Here's how the part is built. I have some questions about the finished solid (model axes, mm). A direction names the side the tool comes from. Coordinates: 2 decimals unless noted, no trailing zeros. Order: outer loops, then holes, each group sorted by start corner. A loop starts at its lowest first (then second) coordinate and runs counter-clockwise, first axis right, second up. Notation, with made-up numbers: (-27.5, -32.75) - (-9.5, -32.75) arc R7 ccw to (-9.5, -21.75) - close; hole circle Ø9 at (89.5, 31). An arc over 180 degrees is marked (long way). Answer as CSV lines item,"result". Start each with the question number.
Q1. I need wall thicknesses on line 1 (Z direction, x = 0, y = 63); line 2 (Y direction, x = -1.25, z = -1). Which ranges of each line are inside material? Lowest first, please.
Q2. Suppose I cut it at C-C (y = 25). Please give me the cut outline in (x, z).
Q3. Suppose I cut it at A-A (y = 59.5). Please give me the cut outline in (x, z), then the cut area to 3 significant figures.
Q4. For pin 1 Ø2 at (y, z) = (73, -3.5) entering from -X; pin 2 Ø2 at (x, y) = (4, 76.5) entering from -Z; pin 3 Ø2 at (y, z) = (88.5, -2.5) entering from -X, each with a flat end and sliding along its axis, tell me the tip position at first contact or that it passes through.
Q5. Thinking about a two-plate mould opening in Z: for faces 4 (the face through (-5.05, 4.93, -2.86)), 5 (the face through (-2.35, 5.028, -1.325)), 6 (the face through (3.5, 86, 2.1)), 7 (the face through (5.05, 86.91, 2.86)), which applies, released by +Z, released by -Z, zero draft, split by the parting line, or undercut?
Q6. For faces 1 (the face through (4.44, 92.1, -2.61)), 2 (the face through (0, 85, -5.802)), 3 (the face through (-1.19, 44.02, -5.37)), which set-ups out of +Z, -Z, +X, -X, +Y, -Y let a thin tool reach every point of the face, with its end or its side?
Q7. Suppose I cut it at B-B (z = -4). Please give me the cut outline in (x, y), then the cut area to 3 significant figures.
Autodesk Inventor part; units mm, degrees
ref_plane "YZ Plane" through (0, 0, 0) normal (1, 0, 0) x (0, 1, 0)
ref_plane "XZ Plane" through (0, 0, 0) normal (0, 1, 0) x (-1, 0, 0)
ref_plane "XY Plane" through (0, 0, 0) normal (0, 0, 1) x (1, 0, 0)
sketch "スケッチ1" plane through (0, 0, 0) normal (0, 1, 0) x (-1, 0, 0)
  line L0 (6.7, 0) -> (3.35, -5.8024)
  line L1 (3.35, -5.8024) -> (-3.35, -5.8024)
  line L2 (-3.35, -5.8024) -> (-6.7, 0)
  line L3 (-6.7, 0) -> (-3.35, 5.8024)
  line L4 (-3.35, 5.8024) -> (3.35, 5.8024)
  line L5 (3.35, 5.8024) -> (6.7, 0)
  point P0 (0, 0)
  point P1 (0, 0)
  dimension "d0" = 6.7
extrude "押し出し1" add sketch "スケッチ1" along normal blind 10
sketch "スケッチ2" plane through (0, 10, 0) normal (0, 1, 0) x (1, 0, 0)
  circle A0 centre (0, 0) radius 5.5
  dimension "d3" = 11
extrude "押し出し2" add sketch "スケッチ2" along normal blind 69
sketch "スケッチ3" plane through (0, 79, 0) normal (0, 1, 0) x (1, 0, 0)
  line L0 (-6.7, 0) -> (-3.35, 5.8024)
  line L1 (-3.35, 5.8024) -> (3.35, 5.8024)
  line L2 (3.35, 5.8024) -> (6.7, 0)
  line L3 (6.7, 0) -> (3.35, -5.8024)
  line L4 (3.35, -5.8024) -> (-3.35, -5.8024)
  line L5 (-3.35, -5.8024) -> (-6.7, 0)
  point P0 (0, 0)
  point P1 (0, 0)
extrude "押し出し3" add sketch "スケッチ3" along normal blind 13.1
sketch "スケッチ4" plane through (0, 92.1, 0) normal (0, 1, 0) x (1, 0, 0)
  circle A0 centre (0, 0) radius 5
  dimension "d8" = 10
extrude "押し出し4" add sketch "スケッチ4" along normal blind 8
sketch "スケッチ5" plane through (0, 100.1, 0) normal (0, 1, 0) x (1, 0, 0)
  circle A0 centre (0, 0) radius 2.5
  dimension "d11" = 5
extrude "押し出し5" cut sketch "スケッチ5" against normal blind 50
sketch "スケッチ6" plane through (6.7, 0, 0) normal (0.866, 0, 0.5) x (0.5, 0, -0.866)
  line L0 (-3.35, 0) -> (-3.35, 10)
  line L1 (-8.85, 10) -> (2.15, 10)
  point P0 (-3.35, 5)
hole "穴1" at (5.025, 5, 2.9012) direction (-0.866, 0, -0.5) diameter 4 depth 8.5
sketch "スケッチ7" plane through (6.7, 79, 0) normal (0.866, 0, 0.5) x (0.5, 0, -0.866)
  line L0 (0, 0) -> (-6.7, 0)
  line L1 (-3.35, 0) -> (-3.35, 13.1)
  line L2 (-6.7, 13.1) -> (0, 13.1)
  point P0 (-3.35, -79)
  point P1 (-3.35, 5)
  dimension "d21" = 5
hole "穴2" at (5.025, 84, 2.9012) direction (-0.866, 0, -0.5) diameter 4 depth 5
properties part number "SMC_CJ1KB10-45(本体)"
Here are the results:
1,line 1,"z = -5.5 to -2.5, 2.5 to 5.5"
1,line 2,"y = 0 to 3.01, 6.99 to 50.1"
2,outline,"circle Ø11 at (0, 0)"
3,outline,"circle Ø11 at (0, 0); hole circle Ø5 at (0, 0)"
3,area,"75.4 mm²"
4,pin 1,"stops at x = -4.9"
4,pin 2,"stops at z = -4.61"
4,pin 3,"stops at x = -5.83"
5,face 4,"released by -Z"
5,face 5,"undercut"
5,face 6,"undercut"
5,face 7,"released by +Z"
6,face 1,"+Y"
6,face 2,"-Z, +X, -X, +Y, -Y"
6,face 3,"none"
7,outline,"(-4.39, 0) - (4.39, 0) - (4.39, 10) - (3.77, 10) - (3.77, 79) - (4.39, 79) - (4.39, 92.1) - (3, 92.1) - (3, 100.1) - (-3, 100.1) - (-3, 92.1) - (-4.39, 92.1) - (-4.39, 79) - (-3.77, 79) - (-3.77, 10) - (-4.39, 10) - close"
7,area,"772 mm²"
